Autodesk Inventor part; units mm, degrees
ref_plane "YZ Plane" through (0, 0, 0) normal (1, 0, 0) x (0, 1, 0)
ref_plane "XZ Plane" through (0, 0, 0) normal (0, 1, 0) x (-1, 0, 0)
ref_plane "XY Plane" through (0, 0, 0) normal (0, 0, 1) x (1, 0, 0)
sketch "Эскиз1" plane through (0, 0, 0) normal (0, 0, 1) x (1, 0, 0)
  line L0 (19, -8.5) -> (-19, -8.5)
  line L1 (-19, -8.5) -> (-19, 8.5)
  line L2 (-19, 8.5) -> (19, 8.5)
  line L3 (19, 8.5) -> (19, -8.5)
  line L4 (19, -8.5) -> (-19, 8.5) construction
  line L5 (-19, -8.5) -> (19, 8.5) construction
  line L6 (22, -11.5) -> (-22, -11.5)
  line L7 (-22, -11.5) -> (-22, 11.5)
  line L8 (-22, 11.5) -> (22, 11.5)
  line L9 (22, 11.5) -> (22, -11.5)
  line L10 (22, -11.5) -> (-22, 11.5) construction
  line L11 (-22, -11.5) -> (22, 11.5) construction
  point P0 (0, 0)
  dimension "d0" = 44
  dimension "d1" = 23
  dimension "d2" = 3
  dimension "d3" = 3
extrude "Выдавливание1" add sketch "Эскиз1" along normal blind 1
sketch "Эскиз2" plane through (0, 0, 1) normal (0, 0, 1) x (1, 0, 0)
  line L0 (22, 11.5) -> (-22, 11.5)
  line L1 (-22, 11.5) -> (-22, -11.5)
  line L2 (-22, -11.5) -> (22, -11.5)
  line L3 (22, -11.5) -> (22, 11.5)
  line L4 (19, -8.5) -> (-19, -8.5)
  line L5 (-19, -8.5) -> (-19, 8.5)
  line L6 (-19, 8.5) -> (19, 8.5)
  line L7 (19, 8.5) -> (19, -8.5)
  line L8 (-23, 12.5) -> (23, 12.5)
  line L9 (23, 12.5) -> (23, -12.5)
  line L10 (23, -12.5) -> (-23, -12.5)
  line L11 (-23, -12.5) -> (-23, 12.5)
  point P0 (0, 0)
  dimension "d6" = 1
extrude "Выдавливание2" add sketch "Эскиз2" against normal blind 3 contours L8 L9 L10 L11
fillet "Сопряжение1" radius 2 8 edges at (23, 12.5, -0.5) (-23, 12.5, -0.5) (-23, -12.5, -0.5) (23, -12.5, -0.5) (-19, 8.5, 0.5) (19, 8.5, 0.5) (19, -8.5, 0.5) (-19, -8.5, 0.5)
properties part number "крышечка"
Verification items for the finished model (mm, model axes). A direction names the side the tool comes from. Give positions to 0.01 mm unless a question says otherwise; leave off trailing zeros. Order: outer loops, then holes, each group sorted by start corner. A loop starts at its lowest first (then second) coordinate and runs counter-clockwise, first axis right, second up. Notation, with made-up numbers: (-33, 71.25) - (25, 71.25) arc R26 cw to (25, 102.25) - close; hole circle Ø1 at (28.25, -30.75). An arc over 180 degrees is marked (long way). Answer as CSV lines item,"result". Start each with the question number.
Item 1: Mould release check, pull along Y, two halves, no side actions. Record for faces 4 (the face through (-22.4, -11.93, -0.52)), 5 (the face through (-22, 0, -1)), 6 (the face through (22.4, 11.93, -0.52)): released by +Y, released by -Y, zero draft, split by the parting line, or undercut.
Item 2: Material ranges on L1, parallel to X at y = 10.5, z = -1.75; L2, parallel to Y at x = -8, z = -1.2; L3, parallel to Y at x = 13.5, z = 0.4, recorded low to high.
Item 3: Section check C-C, the plane x = -1. Record the boundary of the cut face in (y, z), plus the area to 3 significant figures.
Item 4: Section check D-D, the plane y = -11. Record the boundary of the cut face in (x, z), plus the area to 3 significant figures.
Item 5: Access from +Z, -Z, +X, -X, +Y, -Y to the whole of each face (thin tool, end or side, straight path). Record for faces 1 (the face through (0, -11.5, -1)), 2 (the face through (19, 0.1, 0.5)), 3 (the face through (22.43, -11.9, -0.52)).
Item 6: Section check B-B, the plane z = -0.55. Record the boundary of the cut face in (x, y), plus the area to 3 significant figures.
Item 7: Gauge pin test, flat ends, axial feed: pin 1 (8 mm diameter, centred on x = -11.5, y = 6.5, fed in from +Z); pin 2 (2 mm diameter, centred on x = -14, y = 9, fed in from -Z); pin 3 (7 mm diameter, centred on x = 6, y = -2, fed in from -Z). Record the tip position at first contact, or that the pin passes through.
Item 8: Section check A-A, the plane y = -2.25. Record the boundary of the cut face in (x, z).
Filled in:
1,face 4,"released by -Y"
1,face 5,"undercut"
1,face 6,"released by +Y"
2,L1,"-23 to -22, 22 to 23"
2,L2,"-12.5 to -11.5, 11.5 to 12.5"
2,L3,"-12.5 to -8.5, 8.5 to 12.5"
3,outline,"(-12.5, -2) - (-11.5, -2) - (-11.5, 0) - (-8.5, 0) - (-8.5, 1) - (-12.5, 1) - close; (8.5, 0) - (11.5, 0) - (11.5, -2) - (12.5, -2) - (12.5, 1) - (8.5, 1) - close"
3,area,"12.0 mm^2"
4,outline,"(-22.94, -2) - (-22, -2) - (-22, 0) - (22, 0) - (22, -2) - (22.94, -2) - (22.94, 1) - (-22.94, 1) - close"
4,area,"49.6 mm^2"
5,face 1,"-Z"
5,face 2,"+Z, -Z"
5,face 3,"+Z, -Z, +X, -Y"
6,outline,"(-23, -10.5) arc R2 ccw to (-21, -12.5) - (21, -12.5) arc R2 ccw to (23, -10.5) - (23, 10.5) arc R2 ccw to (21, 12.5) - (-21, 12.5) arc R2 ccw to (-23, 10.5) - close; hole (-22, -11.5) - (22, -11.5) - (22, 11.5) - (-22, 11.5) - close"
6,area,"135 mm^2"
7,pin 1,"z = 1"
7,pin 2,"z = 0"
7,pin 3,"through"
8,outline,"(-23, -2) - (-22, -2) - (-22, 0) - (-19, 0) - (-19, 1) - (-23, 1) - close; (19, 0) - (22, 0) - (22, -2) - (23, -2) - (23, 1) - (19, 1) - close"
